Geometry: final body of the model. Coordinates: model frame, mm. A direction names the side the tool comes from. Round coordinates to 2 decimals unless told otherwise and drop trailing zeros. Order: outer loops, then holes, each group sorted by start corner. A loop starts at its lowest first (then second) coordinate and runs counter-clockwise, first axis right, second up. Notation, with made-up numbers: (79, 52.5) -> (126, 52.5) arc R13 ccw to (126, 61.5) -> close; hole circle Ø5 at (-21, -34). An arc over 180 degrees is marked (long way). Put each result on its own line as item: value.
```python
from build123d import *

# Parameters (mm, degrees)
EXTRUDE_1_DEPTH = 80


with BuildPart() as part:
    # 草图1 → 凸台-拉伸1 (new body)
    with BuildSketch(Plane.XY):
        with BuildLine():
            Line((-4, 18.3), (-4, 14.456832295))
            ThreePointArc((-4, 14.456832295), (0, -15), (4, 14.456832295))
            Line((4, 14.456832295), (4, 18.3))
            Line((4, 18.3), (-4, 18.3))
        make_face()
        with BuildLine():
            Line((-3, 9.539392014), (-3, 12.5))
            Line((-3, 12.5), (3, 12.5))
            Line((3, 12.5), (3, 9.539392014))
            ThreePointArc((3, 9.539392014), (0, -10), (-3, 9.539392014))
        make_face(mode=Mode.SUBTRACT)
    extrude(amount=EXTRUDE_1_DEPTH)


solid = part.part
```
1. Cut plane D-D on y = -11. Return loops of the section in (x, z).
Ans:
outline: (-10.2, 0) -> (10.2, 0) -> (10.2, 80) -> (-10.2, 80) -> close
2. Draft query along Y for faces 1 (the face through (0, -10, 39)), 2 (the face through (-10, 2, 80)), 3 (the face through (-0.603, -14.988, 39.44)), 4 (the face through (0, 12.5, 39)). Return one class per face: +Y half, -Y half, draft (parallel to the pull), parting line (faces both ways), or undercut.
Ans:
face 1: undercut
face 2: draft
face 3: parting line
face 4: undercut
3. Material intervals for probe 1 along X at (y, z) = (0, 60); probe 2 along X at (y, z) = (15, 24); probe 3 along Y at (x, z) = (-8.5, 24.5), sorted ascending.
Ans:
probe 1: -15 to -10, 10 to 15
probe 2: -4 to 4
probe 3: -12.36 to -5.27, 5.27 to 12.36
4. Contact query for flat-ended pins moving along their axis: P1, Ø2, axis at y = 7, z = 60, coming from the -X side; P2, Ø1.2, axis at y = 16, z = 39, coming from the -X side; P3, Ø8, axis at x = -1.5, y = -7, coming from the +Z side; P4, Ø2.5, axis at y = 11.5, z = 42, coming from the +X side. Output: stop coordinate, or through.
Ans:
P1: x = -13.75
P2: x = -4
P3: z = 80
P4: x = 10.95
5. Set-up query: faces 5 (the face through (-4, 16, 39)), 6 (the face through (-3, 11, 39)), 7 (the face through (4, 16, 39)). Return all of +Z, -Z, +X, -X, +Y, -Y with unobstructed straight access to the full face (end or side cutting, diameter ignored); none if empty.
Ans:
face 5: +Z, -Z, -X, +Y
face 6: +Z, -Z
face 7: +Z, -Z, +X, +Y
6. Cut plane A-A on y = 0. Return loops of the section in (x, z), and give its area (3 significant figures).
Ans:
outline: (-15, 0) -> (-10, 0) -> (-10, 80) -> (-15, 80) -> close; (10, 0) -> (15, 0) -> (15, 80) -> (10, 80) -> close
area: 800 mm²
7. Cut plane B-B on z = 51.5. Return loops of the section in (x, y), and give its area (3 significant figures).
Ans:
outline: (-4, 14.46) arc R15 ccw (long way) to (4, 14.46) -> (4, 18.3) -> (-4, 18.3) -> close; hole (-3, 9.54) arc R10 ccw (long way) to (3, 9.54) -> (3, 12.5) -> (-3, 12.5) -> close
area: 405 mm²
8. Cut plane C-C on x = 0. Return loops of the section in (y, z), and give its area (3 significant figures).
Ans:
outline: (-15, 0) -> (-10, 0) -> (-10, 80) -> (-15, 80) -> close; (12.5, 0) -> (18.3, 0) -> (18.3, 80) -> (12.5, 80) -> close
area: 864 mm²
